Build history of the part. All positions in model axes, mm. Round coordinates to 2 decimals unless told otherwise and drop trailing zeros. Write each loop counter-clockwise with the first axis right and the second up, starting at its lowest first coordinate (ties: lowest second). Pieces come first, ordered by that corner, then holes. Notation, with made-up numbers: (-22.75, -2.75) -> (-3.75, -2.75) arc R36 ccw to (-3.75, 31.25) -> close; hole circle Ø7 at (20.25, 76.25). An arc over 180 degrees is marked (long way). One line per question, with ' | ' between items.
from build123d import *

# Parameters (mm, degrees)
EXTRUDE_1_DEPTH     = 3
SKETCH_2_R          = 1.6
SKETCH_2_R_2        = 2.1
CUT_EXTRUDE_1_DEPTH = 47.19523785


with BuildPart() as part:
    # 草图1 → 凸台-拉伸1 (new body)
    with BuildSketch(Plane.XY):
        Polygon((0, 0), (10, 0), (30, -20), (30, -35), (-20, -35), (-20, -20), align=None)
    extrude(amount=EXTRUDE_1_DEPTH)

    # 草图2 → 切除-拉伸1 (cut, through all)
    with BuildSketch(Plane.XY.offset(3)):
        with Locations((-15, -31.25)):
            Circle(SKETCH_2_R)
        with Locations(Location((-5, -31.25, 0), (0, 0, 180))):
            Circle(SKETCH_2_R)
        with Locations((-5, -23.75)):
            Circle(SKETCH_2_R)
        with Locations(Location((-15, -23.75, 0), (0, 0, 180))):
            Circle(SKETCH_2_R)
        with Locations((25, -23.75)):
            Circle(SKETCH_2_R)
        with Locations(Location((15, -23.75, 0), (0, 0, 180))):
            Circle(SKETCH_2_R)
        with Locations((15, -31.25)):
            Circle(SKETCH_2_R)
        with Locations(Location((25, -31.25, 0), (0, 0, 180))):
            Circle(SKETCH_2_R)
        with Locations((5, -5)):
            Circle(SKETCH_2_R_2)
        with Locations((5, -15)):
            Circle(SKETCH_2_R_2)
    extrude(amount=-CUT_EXTRUDE_1_DEPTH, mode=Mode.SUBTRACT)


solid = part.part
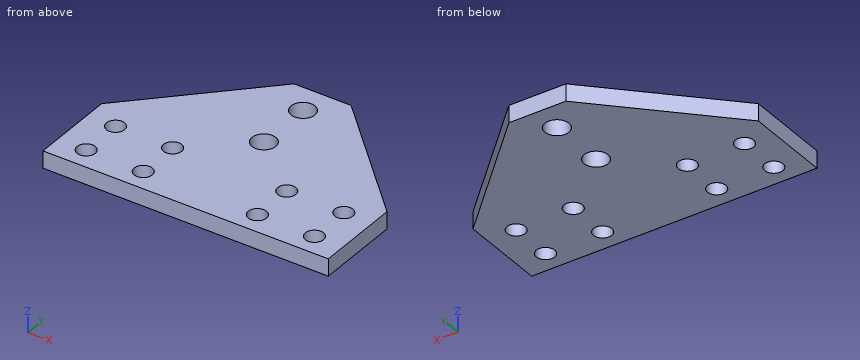
(1) Wall check: line 1 (Y direction, x = 5, z = 0.9); line 2 (Y direction, x = -4, z = 2.6); line 3 (X direction, y = -25, z = 0.9). Give the ranges that are in metal, low to high. Write a range as from..to.
Calculated:
line 1: -35..-17.1, -12.9..-7.1, -2.9..0 | line 2: -35..-32.5, -30..-25, -22.5..-4 | line 3: -20..-16, -14..-6, -4..14, 16..24, 26..30
(2) Drop a flat-ended pin along its axis: pin 1 (3 mm diameter, centred on x = -5, y = -31.25, fed in from -Z). Give the stop position or say it passes through.
Calculated:
pin 1: through
(3) Slice it at B-B (z = 0.8). State how many separate pieces and enclosed holes the cut face has, then the cut area to 3 significant figures.
Calculated:
separate pieces: 1 | enclosed holes: 10 | area: 1,260 mm2
(4) Slice it at C-C (x = -15). Write the cut outline in (y, z), then the cut area to 3 significant figures.
Calculated:
outline: (-35, 0) -> (-32.85, 0) -> (-32.85, 3) -> (-35, 3) -> close; (-29.65, 0) -> (-25.35, 0) -> (-25.35, 3) -> (-29.65, 3) -> close; (-22.15, 0) -> (-15, 0) -> (-15, 3) -> (-22.15, 3) -> close | area: 40.8 mm2
(5) Slice it at D-D (y = -15). Write the cut outline in (x, z), then the cut area to 3 significant figures.
Calculated:
outline: (-15, 0) -> (2.9, 0) -> (2.9, 3) -> (-15, 3) -> close; (7.1, 0) -> (25, 0) -> (25, 3) -> (7.1, 3) -> close | area: 107 mm2
(6) Slice it at A-A (y = -5). Write the cut outline in (x, z).
Calculated:
outline: (-5, 0) -> (2.9, 0) -> (2.9, 3) -> (-5, 3) -> close; (7.1, 0) -> (15, 0) -> (15, 3) -> (7.1, 3) -> close
